from build123d import *

# Parameters (mm, degrees)
F1_DEPTH = 25.4
F3_DEPTH = 22.86
F4_W     = 10.16
F4_H     = 1.748005039
F5_DEPTH = 22.86


with BuildPart() as f1:
    # F0 (on Top) → F1 (new body)
    with BuildSketch(Plane.XY):
        Polygon((-11.43, -15.732045351), (11.43, -15.732045351), (18.4941284914, 6.0091066115), (0, 19.4458774789), (-18.4941284914, 6.0091066115), align=None)
    extrude(amount=F1_DEPTH)

    # F2 (on Top) → F3 (cut)
    with BuildSketch(Plane.XY):
        Polygon((10.16, -13.984040312), (16.4392253257, 5.3414280991), (0, 17.2852244257), (-16.4392253257, 5.3414280991), (-10.16, -13.984040312), align=None)
    extrude(amount=F3_DEPTH, mode=Mode.SUBTRACT)

    # F4 (on face) → F5 (cut)
    with BuildSketch(Plane(origin=(0, 0, 0), x_dir=(1, 0, 0), z_dir=(0, 0, -1))):
        Polygon((-14.8694189943, -0.5100609964), (-13.2996126628, 4.3213061064), (-14.9620642457, 4.8614693697), (-16.5318705771, 0.030102267), align=None)
        Polygon((-14.9620642457, 4.8614693697), (-13.2996126628, 4.3213061064), (-11.7298063314, 9.1526732092), (-13.3922579143, 9.6928364725), align=None)
        Polygon((11.7298063314, 9.1526732092), (13.2996126628, 4.3213061064), (14.9620642457, 4.8614693697), (13.3922579143, 9.6928364725), align=None)
        Polygon((14.9620642457, 4.8614693697), (13.2996126628, 4.3213061064), (14.8694189943, -0.5100609964), (16.5318705771, 0.030102267), align=None)
        Polygon((0, -19.4458774789), (0, -17.2852244257), (-5.08, -13.5943883834), (-5.08, -15.7550414367), align=None)
        Polygon((5.08, -13.5943883834), (0, -17.2852244257), (0, -19.4458774789), (5.08, -15.7550414367), align=None)
        with Locations((0, 14.8580428315)):
            Rectangle(F4_W, F4_H)
    extrude(amount=-F5_DEPTH, mode=Mode.SUBTRACT)


solid = f1.part
Work out the finished part from the listing and answer in its coordinate system (mm). A direction names the side the tool comes from. Give positions to 0.01 mm unless a question says otherwise; leave off trailing zeros. Write each loop counter-clockwise with the first axis right and the second up, starting at its lowest first coordinate (ties: lowest second). Pieces come first, ordered by that corner, then holes.
Q1. The part is cut by section D-D on y = -6.5. Give the vertices of the cut face in (x, z), and give its area (3 significant figures).
Answer:
outline: (-14.43, 22.86) - (14.43, 22.86) - (14.43, 25.4) - (-14.43, 25.4) - close
area: 73.3 mm2
Q2. Given pin 1 (10 mm diameter, centred on x = -7, y = 5.5, fed in from -Z); pin 2 (5 mm diameter, centred on x = -2.5, z = 16.5, fed in from +Y); pin 3 (0.5 mm diameter, centred on y = -15, z = 15, fed in from +X); pin 4 (4 mm diameter, centred on x = -7, z = 8, fed in from +Y), each flat-ended and moving along its own axis, determine where each tip first touches the part or whether it passes through.
Answer:
pin 1: stops at z = 22.86
pin 2: passes through
pin 3: stops at x = 11.75
pin 4: stops at y = 15.76
Q3. Straight lines are drawn through the part: L1, parallel to Z at x = 3, y = -3.5; L2, parallel to X at y = -10.5, z = 13.75; L3, parallel to X at y = 10, z = 11. For each, find the intervals that lie inside material, in ascending order.
Answer:
L1: z = 22.86 to 25.4
L2: x = -13.13 to -11.29, 11.29 to 13.13
L3: x = -13 to -10.03, 10.03 to 13
Q4. For a pull along X with two mould halves and no side action, classify faces 1 (the face through (-5.08, -15, 11)), 2 (the face through (10.4, -13.9, 0)), 3 (the face through (12.573, -9.427, 11.27)) as released by +X, released by -X, zero draft, split by the parting line, or undercut.
Answer:
face 1: undercut
face 2: zero draft
face 3: released by +X
Q5. The part is cut by section C-C on y = 11.5. Give the vertices of the cut face in (x, z).
Answer:
outline: (-10.94, 0) - (-7.96, 0) - (-7.96, 22.86) - (7.96, 22.86) - (7.96, 0) - (10.94, 0) - (10.94, 25.4) - (-10.94, 25.4) - close
Q6. The part is cut by section B-B on x = -7. Give the vertices of the cut face in (y, z), and give its area (3 significant figures).
Answer:
outline: (-15.73, 0) - (-13.98, 0) - (-13.98, 22.86) - (12.2, 22.86) - (12.2, 0) - (14.36, 0) - (14.36, 25.4) - (-15.73, 25.4) - close
area: 166 mm2
Q7. A tool of negligible diameter and unlimited length cuts with its end or side. For faces 4 (the face through (-12.55, -9.42, 11.27)), 5 (the face through (-8, -13.984, 11)), 6 (the face through (-10.5, -13.9, 0)), 7 (the face through (-15.712, 0.236, 11.27)), 8 (the face through (5.08, 15, 11)), from which of +Z, -Z, +X, -X, +Y, -Y can it reach the whole face along a straight path? Write none if from no direction.
Answer:
face 4: -Z, -X
face 5: -Z
face 6: -Z, +X, -X, +Y, -Y
face 7: -Z, -Y
face 8: -Z, +Y, -Y
Q8. The part is cut by section A-A on z = 3. Give the vertices of the cut face in (x, y).
Answer:
outline: (-18.49, 6.01) - (-16.53, -0.03) - (-14.87, 0.51) - (-16.44, 5.34) - (-5.08, 13.59) - (-5.08, 15.76) - close; (-13.39, -9.69) - (-11.43, -15.73) - (-5.08, -15.73) - (-5.08, -13.98) - (-10.16, -13.98) - (-11.73, -9.15) - close; (5.08, -15.73) - (11.43, -15.73) - (13.39, -9.69) - (11.73, -9.15) - (10.16, -13.98) - (5.08, -13.98) - close; (5.08, 13.59) - (16.44, 5.34) - (14.87, 0.51) - (16.53, -0.03) - (18.49, 6.01) - (5.08, 15.76) - close
